```python
from build123d import *

# Parameters (mm, degrees)
SKETCH_1_R          = 13.6
SKETCH_1_R_2        = 12.45
EXTRUDE_1_DEPTH     = 20
SKETCH_2_R          = 20
EXTRUDE_2_DEPTH     = 5
SKETCH_3_R          = 13.1
CUT_EXTRUDE_1_DEPTH = 2.5
SKETCH_4_R          = 12.45
CUT_EXTRUDE_2_DEPTH = 10


with BuildPart() as part:
    # 草图1 → 凸台-拉伸1 (new body)
    with BuildSketch(Plane(origin=(0, 0, 0), x_dir=(1, 0, 0), z_dir=(0, 1, 0))):
        with Locations(Location((0, 0, 0), (0, 0, 270))):
            Circle(SKETCH_1_R)
        with Locations(Location((0, 0, 0), (0, 0, 270))):
            Circle(SKETCH_1_R_2, mode=Mode.SUBTRACT)
    extrude(amount=EXTRUDE_1_DEPTH)

    # 草图2 → 凸台-拉伸2 (add)
    with BuildSketch(Plane(origin=(0, 20, 0), x_dir=(1, 0, 0), z_dir=(0, 1, 0))):
        with Locations(Location((0, 0, 0), (0, 0, 270))):
            Circle(SKETCH_2_R)
    extrude(amount=-EXTRUDE_2_DEPTH)

    # 草图3 → 切除-拉伸1 (cut)
    with BuildSketch(Plane(origin=(0, 20, 0), x_dir=(1, 0, 0), z_dir=(0, 1, 0))):
        with Locations(Location((0, 0, 0), (0, 0, 270))):
            Circle(SKETCH_3_R)
    extrude(amount=-CUT_EXTRUDE_1_DEPTH, mode=Mode.SUBTRACT)

    # 草图4 → 切除-拉伸2 (cut)
    with BuildSketch(Plane.XZ.offset(-15)):
        with Locations(Location((0, 0, 0), (0, 0, 90))):
            Circle(SKETCH_4_R)
    extrude(amount=-CUT_EXTRUDE_2_DEPTH, mode=Mode.SUBTRACT)

    # 草图5 → 切除-旋转2 (revolve, cut)
    with BuildSketch(Plane(origin=(0, 0, 0), x_dir=(0, 0, -1), z_dir=(1, 0, 0))):
        Polygon((20, 17), (13.6, 15), (20, 15), align=None)
    revolve(axis=Axis((0, 0, 0), (0, 1, 0)), mode=Mode.SUBTRACT)


solid = part.part
```
Input: part model. Units: mm. Frame: model coordinates. A direction names the side the tool comes from. Coordinates: 2 decimals unless noted, no trailing zeros. Write each loop counter-clockwise with the first axis right and the second up, starting at its lowest first coordinate (ties: lowest second). Pieces come first, ordered by that corner, then holes. Notation, with made-up numbers: M 36,55 L 75,55 A11 ccw 75,70 Z; hole C -30,76 d3. An arc over 180 degrees is marked long. Use one line per item in the form item = value.
Q1. Material intervals for probe 1 along X at (y, z) = (18.5, 0); probe 2 along X at (y, z) = (9, -5.5); probe 3 along Z at (x, y) = (-7, 3), sorted ascending. Write a range as from..to.
Answer below:
probe_1 = -20..-13.1, 13.1..20
probe_2 = -12.44..-11.17, 11.17..12.44
probe_3 = -11.66..-10.3, 10.3..11.66
Q2. Section A-A (z = 0). Return loops of the section in (x, y).
Answer below:
outline = M -20,17 L -13.6,15 L -13.6,0 L -12.45,0 L -12.45,17.5 L -13.1,17.5 L -13.1,20 L -20,20 Z; M 12.45,0 L 13.6,0 L 13.6,15 L 20,17 L 20,20 L 13.1,20 L 13.1,17.5 L 12.45,17.5 Z
Q3. Section B-B (x = 0). Return loops of the section in (y, z), plus the area to 4 significant figures.
Answer below:
outline = M 0,-13.6 L 15,-13.6 L 17,-20 L 20,-20 L 20,-13.1 L 17.5,-13.1 L 17.5,-12.45 L 0,-12.45 Z; M 0,12.45 L 17.5,12.45 L 17.5,13.1 L 20,13.1 L 20,20 L 17,20 L 15,13.6 L 0,13.6 Z
area = 93.95 mm²
Q4. First-contact query: pin 1 (5 mm diameter, centred on x = 5, y = 11, fed in from +Z); pin 2 (22.5 mm diameter, centred on x = 0, z = 0, fed in from +Y); pin 3 (5 mm diameter, centred on y = 3, z = 5, fed in from -X); pin 4 (4 mm diameter, centred on y = 17.5, z = 9.5, fed in from +X). Flat tips, straight axial feed; report the tip coordinate or a pass-through.
Answer below:
pin_1 = 13.37
pin_2 = through
pin_3 = -13.37
pin_4 = 18.54
Q5. Draft query along X for faces 1 (the face through (-12, 0, 4)), 2 (the face through (11.046, 18.768, 7.042)), 3 (the face through (-19.524, 18.521, -4.336)), 4 (the face through (-12.6, 17.5, -0.1)). Return one class per face: released by +X, released by -X, zero draft, split by the parting line, or undercut.
Answer below:
face_1 = zero draft
face_2 = undercut
face_3 = split by the parting line
face_4 = undercut
Q6. Section C-C (y = 10). Return loops of the section in (x, z).
Answer below:
outline = C 0,0 d27.2; hole C 0,0 d24.9
Q7. Set-up query: faces 5 (the face through (-13.277, 7.395, -2.948)), 6 (the face through (-4, 20, 13)). Return all of +Z, -Z, +X, -X, +Y, -Y with unobstructed straight access to the full face (end or side cutting, diameter ignored); none if empty.
Answer below:
face_5 = -Y
face_6 = +Z, -Z, +X, -X, +Y
